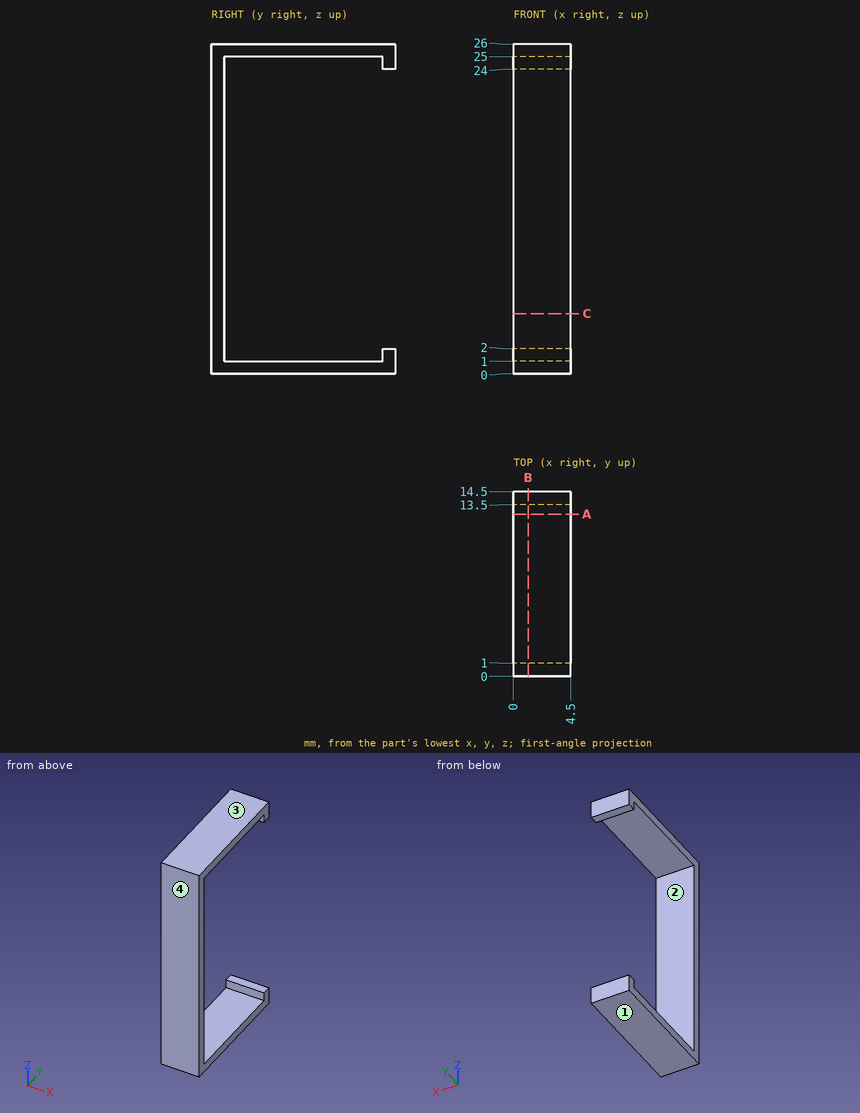
Verification items for this drawing (mm, ordinates from the low corner). Coordinates: 2 decimals unless noted, no trailing zeros. Loops run counter-clockwise (first coordinate to the right, second up) from the corner with the lowest first, then second, coordinate; pieces in that order, holes last. Notation, with made-up numbers: (-9, 73.25) - (38, 73.25) arc R15 ccw to (38, 83.25) - close; hole circle Ø1 at (46.5, 42). An arc over 180 degrees is marked (long way). Use one line per item in the form item = value. Start each with the question number.
Item 1: Mould release check, pull along Z, two halves, no side actions. Record for the marked faces 1, 2, 3 and 4: +Z half, -Z half, draft (parallel to the pull), parting line (faces both ways), or undercut.
Item 2: Section check C-C, the plane z = 4.75. Enter the section's corners in (x, y), and give its area (3 significant figures).
Item 3: Section check A-A, the plane y = 12.75. Enter the section's corners in (x, z), and give its area (3 significant figures).
Item 4: Gauge pin test, flat ends, axial feed: pin 1 (1.3 mm diameter, centred on x = 2.5, z = 10, fed in from +Y); pin 2 (1.3 mm diameter, centred on x = 3, y = 5, fed in from -Z). Record the tip position at first contact, or that the pin passes through.
Item 5: Thickness scan on probe 1 along Z at (x, y) = (2.65, 9); probe 2 along Y at (x, z) = (2.35, 9.25). Record the ranges inside material, lowest first.
Item 6: Section check B-B, the plane x = 1.15. Enter the section's corners in (y, z).
Computed:
q1.face_1 = -Z half
q1.face_2 = undercut
q1.face_3 = +Z half
q1.face_4 = draft
q2.outline = (0, 0) - (4.5, 0) - (4.5, 1) - (0, 1) - close
q2.area = 4.50 mm2
q3.outline = (0, 0) - (4.5, 0) - (4.5, 1) - (0, 1) - close; (0, 25) - (4.5, 25) - (4.5, 26) - (0, 26) - close
q3.area = 9.00 mm2
q4.pin_1 = 1
q4.pin_2 = 0
q5.probe_1 = 0 to 1, 25 to 26
q5.probe_2 = 0 to 1
q6.outline = (0, 0) - (14.5, 0) - (14.5, 2) - (13.5, 2) - (13.5, 1) - (1, 1) - (1, 25) - (13.5, 25) - (13.5, 24) - (14.5, 24) - (14.5, 26) - (0, 26) - close
